from build123d import *

# Parameters (mm, degrees)
F1_DEPTH = 63.5
F2_DEPTH = 25.4
F3_DEPTH = 7.9375
F5_R     = 6.35


with BuildPart() as f1:
    # F0 (on Front) → F1 (new body, symmetric)
    with BuildSketch(Plane.XZ):
        Polygon((-41.275, -9.525), (41.275, -9.525), (41.275, 9.525), (22.225, 9.525), (-41.275, 9.525), align=None)
    extrude(amount=F1_DEPTH, both=True)

    # F0 (on Front) → F2 (join, symmetric)
    with BuildSketch(Plane.XZ):
        with BuildLine():
            Line((22.225, 9.525), (41.275, 9.525))
            Line((41.275, 9.525), (41.275, 33.3553104297))
            ThreePointArc((41.275, 33.3553104297), (44.063311099, 40.086888901), (50.7948895703, 42.8752))
            Line((50.7948895703, 42.8752), (55.4659834841, 42.8752))
            Line((55.4659834841, 42.8752), (55.4659834841, 61.9252))
            Line((55.4659834841, 61.9252), (50.7948895703, 61.9252))
            ThreePointArc((50.7948895703, 61.9252), (30.5929269174, 53.5572730826), (22.225, 33.3553104297))
            Line((22.225, 33.3553104297), (22.225, 9.525))
        make_face()
        Polygon((70.8683976346, 61.9252), (55.4659834841, 61.9252), (55.4659834841, 42.8752), (55.4659834841, 42.8555016406), (80.8659834841, 42.748387903), (80.8659834841, 61.9252), align=None)
    extrude(amount=F2_DEPTH, both=True)

    # F0 (on Front) → F3 (join, symmetric)
    with BuildSketch(Plane.XZ):
        with BuildLine():
            add(Edge.make_bspline(
                [(-41.275, 9.525), (-40.730714798, 32.5702540576), (17.2467883676, 62.170214951), (50.7948895703, 61.9252)],
                knots=[0, 0, 0, 0, 105.9369884673, 105.9369884673, 105.9369884673, 105.9369884673], degree=3))
            Line((-41.275, 9.525), (22.225, 9.525))
            Line((22.225, 9.525), (22.225, 33.3553104297))
            ThreePointArc((22.225, 33.3553104297), (30.5929269174, 53.5572730826), (50.7948895703, 61.9252))
        make_face()
    extrude(amount=F3_DEPTH, both=True)

    # F0 (on Front) → F4 (revolve)
    with BuildSketch(Plane.XZ):
        Polygon((80.8659834841, 61.9252), (80.8659834841, 42.748387903), (80.8659834841, 38.1), (106.2659834841, 38.1), (106.2659834841, 66.675), (80.8659834841, 66.675), align=None)
    revolve(axis=Axis((80.8659834841, 0, 52.3875), (0, 0, -1)))

    # F5
    f5_edges = [f1.edges().sort_by_distance(p)[0] for p in [
        (-41.275, -63.5, 0),
        (41.275, -63.5, 0),
        (41.275, 63.5, 0),
        (-41.275, 63.5, 0),
    ]]
    fillet(f5_edges, radius=F5_R)


solid = f1.part
Input: part model. Units: mm. Frame: model coordinates. A direction names the side the tool comes from. Round coordinates to 2 decimals unless told otherwise and drop trailing zeros. Order: outer loops, then holes, each group sorted by start corner. A loop starts at its lowest first (then second) coordinate and runs counter-clockwise, first axis right, second up. Notation, with made-up numbers: (38.25, 51.5) - (96.25, 51.5) arc R19 cw to (96.25, 73.5) - close; hole circle Ø3 at (14.25, 80). An arc over 180 degrees is marked (long way). Answer as a JSON object with one key per item and string values. Group by question number.
(1) Cut plane C-C (x = 92.5). Return loops of the section in (y, z) (3 decimals), then the cut area to 3 significant figures.
(2) Cut plane A-A (z = -2). Return loops of the section in (x, y) (3 decimals), then the cut area to 3 significant figures.
(3) Reachability of faces 5 (the face through (43.99, -0.36, 40.01)), 6 (the face through (30.82, -16.79, 53.78)), 7 (the face through (22.225, 17, 22)) from +Z, -Z, +X, -X, +Y, -Y: full face, straight path, thin tool, end or side. Return the list, or none.
(4) Pin query (flat end, axial travel): P1, Ø8, axis at x = 21.5, z = 15, coming from the -Y side; P2, Ø10, axis at x = 76, z = 38, coming from the +Y side; P3, Ø13, axis at y = -3, z = 6.5, coming from the +X side (3 decimals). Return the tip coordinate at first contact, or that it passes through.
(5) Cut plane D-D (y = 36.5). Return loops of the section in (x, z) (3 decimals).
(6) Material intervals for probe 1 along Y at (x, z) = (-7, 30.5); probe 2 along Y at (x, z) = (76, 44.5); probe 3 along X at (y, z) = (-29.5, -6) (3 decimals), sorted ascending. Write a range as from..to.
(7) Draft query along X for faces 1 (the face through (45, -25.4, 42)), 2 (the face through (53, 0, 42.875)), 3 (the face through (39.464, 61.59, 0.133)), 4 (the face through (30.82, 16.55, 53.78)). Return one class per face: released by +X, released by -X, zero draft, split by the parting line, or undercut.
Here are the results:
{
 "1": {"outline": "(-22.579, 38.1) - (22.579, 38.1) - (22.579, 66.675) - (-22.579, 66.675) - close", "area": "1,290 mm^2"},
 "2": {"outline": "(-41.275, -57.15) arc R6.35 ccw to (-34.925, -63.5) - (34.925, -63.5) arc R6.35 ccw to (41.275, -57.15) - (41.275, 57.15) arc R6.35 ccw to (34.925, 63.5) - (-34.925, 63.5) arc R6.35 ccw to (-41.275, 57.15) - close", "area": "10,400 mm^2"},
 "3": {"face 5": "-Z, +Y, -Y", "face 6": "+Z, -X, -Y", "face 7": "+Z, -X, +Y"},
 "4": {"P1": "stops at y = -25.4", "P2": "stops at y = 25.4", "P3": "stops at x = 41.275"},
 "5": {"outline": "(-41.275, -9.525) - (41.275, -9.525) - (41.275, 9.525) - (-41.275, 9.525) - close"},
 "6": {"probe 1": "y = -7.94..7.94", "probe 2": "y = -25.4..25.4", "probe 3": "x = -41.275..41.275"},
 "7": {"face 1": "zero draft", "face 2": "undercut", "face 3": "released by +X", "face 4": "released by -X"}
}
